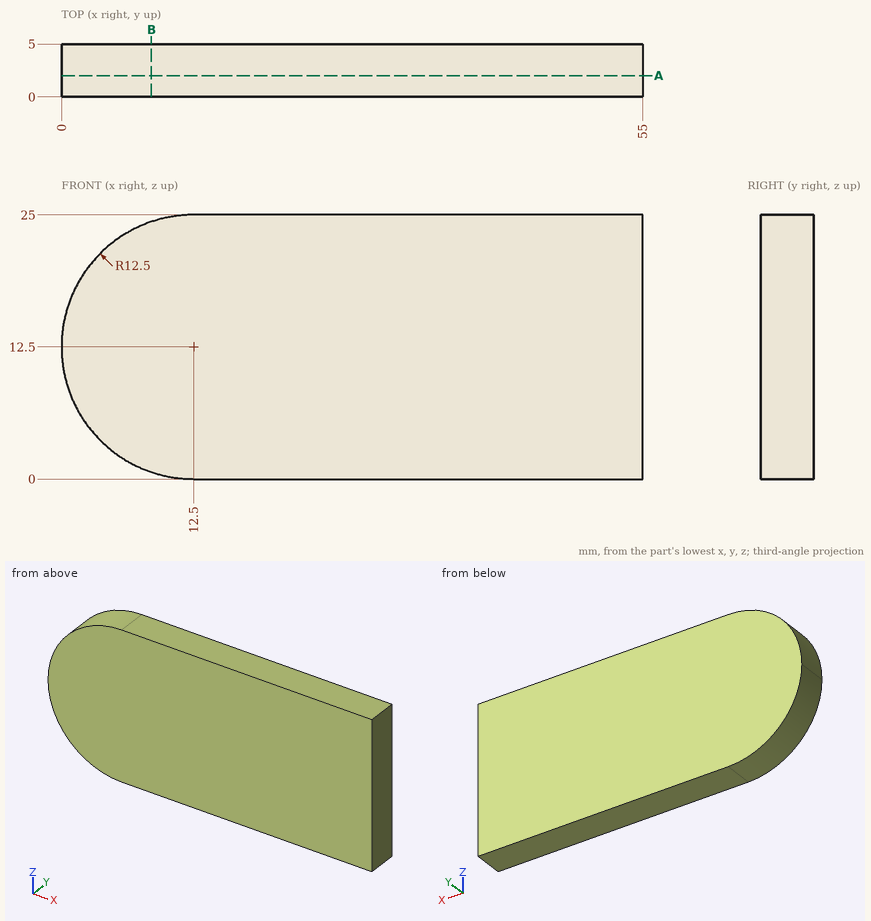
Part print with two shaded views. Sizes in mm from the minimum x, y, z corner. Round coordinates to 2 decimals unless told otherwise and drop trailing zeros. Order: outer loops, then holes, each group sorted by start corner. A loop starts at its lowest first (then second) coordinate and runs counter-clockwise, first axis right, second up. Notation, with made-up numbers: (13.25, 83) -> (47.25, 83) arc R13 ccw to (47.25, 92) -> close; hole circle Ø4 at (59.5, 83.25). An arc over 180 degrees is marked (long way). Use one line per item in the form item = value.
Item 1: Cut at B-B, the plane x = 8.5. Write the cut outline in (y, z), and give its area (3 significant figures).
Returned:
outline = (0, 0.66) -> (5, 0.66) -> (5, 24.34) -> (0, 24.34) -> close
area = 118 mm^2
Item 2: Cut at A-A, the plane y = 2. Write the cut outline in (x, z), and give its area (3 significant figures).
Returned:
outline = (0, 12.5) arc R12.5 ccw to (12.5, 0) -> (55, 0) -> (55, 25) -> (12.5, 25) arc R12.5 ccw to start
area = 1,310 mm^2
Item 3: Drill centre lines: line 1 (Z direction, x = 11, y = 2.25); line 2 (X direction, y = 0.2, z = 21.5); line 3 (Z direction, x = 4.5, y = 3.15). Where is each one in solid material? Low to high.
Returned:
line_1 = 0.09 to 24.91
line_2 = 3.83 to 55
line_3 = 2.9 to 22.1
